The model under review builds one solid part; all positions refer to its coordinate system, in mm. A direction names the side the tool comes from. Give positions to 0.01 mm unless a question says otherwise; leave off trailing zeros. Loops run counter-clockwise (first coordinate to the right, second up) from the corner with the lowest first, then second, coordinate; pieces in that order, holes last. Notation, with made-up numbers: M -32,47 L 15,47 A18 cw 15,62 Z; hole C 13,1.25 d1. An arc over 180 degrees is marked long. Return JSON: item names as keys, results as strings.
Autodesk Inventor part; units mm, degrees
ref_plane "YZ Plane" through (0, 0, 0) normal (1, 0, 0) x (0, 1, 0)
ref_plane "XZ Plane" through (0, 0, 0) normal (0, 1, 0) x (-1, 0, 0)
ref_plane "XY Plane" through (0, 0, 0) normal (0, 0, 1) x (1, 0, 0)
sketch "Sketch1" plane through (0, 0, 0) normal (0, 1, 0) x (-1, 0, 0)
  line L0 (7.5, 7.5) -> (-7.5, 7.5)
  line L1 (-7.5, 7.5) -> (-7.5, -7.5)
  line L2 (-7.5, -7.5) -> (7.5, -7.5)
  line L3 (7.5, -7.5) -> (7.5, 7.5)
  circle A0 centre (0, 0) radius 15
  dimension "d0" = 15
  dimension "d1" = 15
  dimension "d2" = 30
  dimension "d3" = 7.5
  dimension "d4" = 7.5
extrude "Extrusion1" add sketch "Sketch1" along normal blind 5
chamfer "Chamfer1" distance 2 angle 45 2 edges at (15, 5, 0) (15, 0, 0)
properties part number "Test Ring"
1) Consider section C-C on y = 1.35. Write out the cut boundary in (x, z), then the cut area to 3 significant figures.
From the geometry:
{"outline": "C 0,0 d28.7; hole M -7.5,-7.5 L 7.5,-7.5 L 7.5,7.5 L -7.5,7.5 Z", "area": "422 mm²"}
2) Consider section D-D on y = 3.4. Write out the cut boundary in (x, z), then the cut area to 3 significant figures.
From the geometry:
{"outline": "C 0,0 d29.2; hole M -7.5,-7.5 L 7.5,-7.5 L 7.5,7.5 L -7.5,7.5 Z", "area": "445 mm²"}
3) Wall thickness on L1, parallel to X at y = 2.1, z = -0.25; L2, parallel to X at y = 4.55, z = 3; L3, parallel to Z at x = -5, y = 2.5: over which ranges is each line inside the solid? List them lowest first. Write a range as from..to.
From the geometry:
{"L1": "-15..-7.5, 7.5..15", "L2": "-13.11..-7.5, 7.5..13.11", "L3": "-14.14..-7.5, 7.5..14.14"}
4) Insertion check: pin 1 (2.5 mm diameter, centred on y = 2.5, z = 3.5, fed in from +X); pin 2 (2.5 mm diameter, centred on y = 3, z = -2.5, fed in from -X); pin 3 (2 mm diameter, centred on x = 0.5, z = -6, fed in from +Y) (3 decimals). Each pin has a flat end and moves straight along its axis. Give the tip position at first contact, or say it passes through.
From the geometry:
{"pin 1": "x = 14.83", "pin 2": "x = -14.95", "pin 3": "through"}
5) Consider section A-A on z = 0. Write out the cut boundary in (x, y), then the cut area to 3 significant figures.
From the geometry:
{"outline": "M -15,2 L -13,0 L -7.5,0 L -7.5,5 L -13,5 L -15,3 Z; M 7.5,0 L 13,0 L 15,2 L 15,3 L 13,5 L 7.5,5 Z", "area": "67.0 mm²"}
6) Consider section B-B on x = 0. Write out the cut boundary in (y, z).
From the geometry:
{"outline": "M 0,-13 L 2,-15 L 3,-15 L 5,-13 L 5,-7.5 L 0,-7.5 Z; M 0,7.5 L 5,7.5 L 5,13 L 3,15 L 2,15 L 0,13 Z"}
7) The part is to be moulded in two halves that separate along X. For faces 1 (the face through (9.674, 0.125, 8.871)), 2 (the face through (0, 2, 7.5)), 3 (the face through (-8, 5, 0)), say which applies: released by +X, released by -X, zero draft, split by the parting line, or undercut.
From the geometry:
{"face 1": "split by the parting line", "face 2": "undercut", "face 3": "zero draft"}
8) Tool access review of faces 4 (the face through (-8, 0, 0)), 5 (the face through (-7.5, 2, 0)): name each direction out of +Z, -Z, +X, -X, +Y, -Y from which nothing blocks a thin tool from reaching the whole face with its end or side.
From the geometry:
{"face 4": "+Z, -Z, +X, -X, -Y", "face 5": "+Y, -Y"}
